```python
from build123d import *

# Parameters (mm, degrees)
SKETCH1_W           = 210
SKETCH1_H           = 115
BOSS_EXTRUDE2_DEPTH = 30
SKETCH6_W           = 60
SKETCH6_H           = 60
BOSS_EXTRUDE3_DEPTH = 50
SKETCH8_R           = 15
BOSS_EXTRUDE4_DEPTH = 50
FILLET1_R           = 20
BOSS_EXTRUDE5_DEPTH = 80
CUT_EXTRUDE1_DEPTH  = 336.046164359


with BuildPart() as part:
    # Sketch1 → Boss-Extrude2 (new body)
    with BuildSketch(Plane(origin=(0, 0, 0), x_dir=(1, 0, 0), z_dir=(0, 1, 0))):
        Rectangle(SKETCH1_W, SKETCH1_H)
    extrude(amount=BOSS_EXTRUDE2_DEPTH)

    # Sketch6 → Boss-Extrude3 (add, symmetric)
    with BuildSketch(Plane(origin=(0, 0, 0), x_dir=(0, 0, -1), z_dir=(1, 0, 0))):
        with Locations((0, 55.329200869)):
            Rectangle(SKETCH6_W, SKETCH6_H)
    extrude(amount=BOSS_EXTRUDE3_DEPTH, both=True)

    # Sketch8 → Boss-Extrude4 (add, symmetric)
    with BuildSketch(Plane(origin=(0, 0, 0), x_dir=(0, 0, -1), z_dir=(1, 0, 0))):
        with BuildLine():
            Line((40, 295.680123104), (40, 80.041536576))
            ThreePointArc((40, 80.041536576), (0, 72.86082984), (-40, 80.041536576))
            Line((-40, 80.041536576), (-40, 295.680123104))
            ThreePointArc((-40, 295.680123104), (0, 302.86082984), (40, 295.680123104))
        make_face()
        with Locations((0, 270)):
            Circle(SKETCH8_R, mode=Mode.SUBTRACT)
        with Locations((0, 120)):
            Circle(SKETCH8_R, mode=Mode.SUBTRACT)
    extrude(amount=BOSS_EXTRUDE4_DEPTH, both=True)

    # Fillet1
    fillet1_edges = [part.edges().sort_by_distance(p)[0] for p in [
        (-50, 30, 0),
        (0, 30, 30),
        (0, 30, -30),
        (50, 30, 0),
    ]]
    fillet(fillet1_edges, radius=FILLET1_R)

    # Sketch9 → Boss-Extrude5 (add)
    with BuildSketch(Plane(origin=(0, 0, -40), x_dir=(-1, 0, 0), z_dir=(0, 0, -1))):
        Polygon((58, 217.5), (50, 217.5), (50, 194.99999986), (50, 172.5), (58, 172.5), align=None)
    extrude(amount=-BOSS_EXTRUDE5_DEPTH)

    # Sketch9<3> → Cut-Extrude1 (cut, through all)
    with BuildSketch(Plane(origin=(0, 0, -40), x_dir=(-1, 0, 0), z_dir=(0, 0, -1))):
        with BuildLine():
            ThreePointArc((50, 194.999999634), (38.284271377, 223.284271118), (10, 235))
            Line((10, 235), (-50, 235))
            Line((-50, 235), (-50, 155))
            Line((-50, 155), (10, 155))
            ThreePointArc((10, 155), (38.284271118, 166.715728623), (50, 194.999999634))
        make_face()
    extrude(amount=-CUT_EXTRUDE1_DEPTH, mode=Mode.SUBTRACT)


solid = part.part
```
Can you work these out from the model? Positions are in its coordinate system, mm. A direction names the side the tool comes from. Coordinates: 2 decimals unless noted, no trailing zeros. Order: outer loops, then holes, each group sorted by start corner. A loop starts at its lowest first (then second) coordinate and runs counter-clockwise, first axis right, second up.
1. I need wall thicknesses on line 1 (Y direction, x = 15, z = 0); line 2 (Y direction, x = -28.5, z = -10); line 3 (X direction, y = 128, z = -13.5). Which ranges of each line are inside material? Lowest first, please.
2. If we section it at D-D (y = 111.5): Please give me the cut outline in (x, z), then the cut area to 3 significant figures.
3. I'm going to push flat-ended pins straight in: pin 1 (6 mm diameter, centred on y = 67, z = 8.5, fed in from +X); pin 2 (4 mm diameter, centred on y = 210, z = -16, fed in from +X); pin 3 (13.5 mm diameter, centred on x = 5.5, y = 58, fed in from -Z); pin 4 (24 mm diameter, centred on y = 120, z = 0, fed in from -X). Where does each tip first touch, or does it pass through?
4. If we section it at C-C (z = 0): Please give me the cut outline in (x, y), then the cut area to 3 significant figures.
5. For faces 1 (the face through (1, 63, -30)), 2 (the face through (-0.98, 36.014, 35.703)), 3 (the face through (20, 235, -1)), which set-ups out of +Z, -Z, +X, -X, +Y, -Y let a thin tool reach every point of the face, with its end or its side?
6. If we section it at A-A (y = 270): Please give me the cut outline in (x, z), then the cut area to 3 significant figures.
7. Thinking about a two-plate mould opening in Z: for faces 4 (the face through (-54, 217.5, -1)), 5 (the face through (-0.7, 134.872, 1.953)), 6 (the face through (-1, 15, -57.5)), 7 (the face through (-39, 162, 40)), which applies, +Z half, -Z half, draft (parallel to the pull), parting line (faces both ways), or undercut?
8. If we section it at B-B (x = -14.5): Please give me the cut outline in (y, z), then the cut area to 3 significant figures.
Entries:
1. line 1: y = 0 to 105, 135 to 155, 235 to 255, 285 to 302.86
1. line 2: y = 0 to 108.82, 131.18 to 159.54, 230.46 to 258.82, 281.18 to 302.43
1. line 3: x = -50 to 50
2. outline: (-50, -40) - (50, -40) - (50, -12.36) - (-50, -12.36) - close; (-50, 12.36) - (50, 12.36) - (50, 40) - (-50, 40) - close
2. area: 5,530 mm2
3. pin 1: stops at x = 50
3. pin 2: stops at x = -46.21
3. pin 3: stops at z = -30
3. pin 4: passes through
4. outline: (-105, 0) - (105, 0) - (105, 30) - (70, 30) arc R20 cw to (50, 50) - (50, 105) - (-50, 105) - (-50, 50) arc R20 cw to (-70, 30) - (-105, 30) - close; (-58, 172.5) - (-50, 172.5) - (-50, 135) - (50, 135) - (50, 155) - (-10, 155) arc R40 cw to (-10, 235) - (50, 235) - (50, 255) - (-50, 255) - (-50, 217.5) - (-58, 217.5) - close; (-50, 285) - (50, 285) - (50, 302.86) - (-50, 302.86) - close
4. area: 20,800 mm2
5. face 1: -Z, +X, -X
5. face 2: +Z, +X, -X
5. face 3: +Z, -Z, +X
6. outline: (-50, -40) - (50, -40) - (50, -15) - (-50, -15) - close; (-50, 15) - (50, 15) - (50, 40) - (-50, 40) - close
6. area: 5,000 mm2
7. face 4: draft
7. face 5: undercut
7. face 6: -Z half
7. face 7: +Z half
8. outline: (0, -57.5) - (30, -57.5) - (30, -50) arc R20 cw to (50, -30) - (76.84, -30) arc R115 ccw to (80.04, -40) - (155.25, -40) - (155.25, 40) - (80.04, 40) arc R115 ccw to (76.84, 30) - (50, 30) arc R20 cw to (30, 50) - (30, 57.5) - (0, 57.5) - close; (234.75, -40) - (295.68, -40) arc R115 ccw to (295.68, 40) - (234.75, 40) - close; hole circle Ø30 at (120, 0); hole circle Ø30 at (270, 0)
8. area: 16,500 mm2
